from build123d import *

# Parameters (mm, degrees)
SKETCH1_W               = 44.5
SKETCH1_H               = 35
BOSS_EXTRUDE1_DEPTH     = 4
BOSS_EXTRUDE2_DEPTH     = 19.6
SKETCH4_W               = 26
SKETCH4_H               = 31
CUT_EXTRUDE1_DEPTH      = 4
BOSS_EXTRUDE3_DEPTH     = 4
CHAMFER1_SIZE           = 5
CUT_EXTRUDE2_DEPTH      = 62.336856783
CUT_EXTRUDE2_DEPTH_BACK = 62.336856783
SKETCH6_R               = 1.25
SKETCH7_R               = 2.5
SKETCH7_R_2             = 1.25
BOSS_EXTRUDE4_DEPTH     = 4
FILLET1_R               = 0.5
FILLET3_R               = 0.25
CUT_EXTRUDE3_DEPTH      = 60.911685095
CUT_EXTRUDE3_DEPTH_BACK = 60.911685095
SKETCH8_R               = 1.25


with BuildPart() as part:
    # Sketch1 → Boss-Extrude1 (new body)
    with BuildSketch(Plane(origin=(0, 0, 0), x_dir=(1, 0, 0), z_dir=(0, 1, 0))):
        with Locations((22.25, 17.5)):
            Rectangle(SKETCH1_W, SKETCH1_H)
    extrude(amount=BOSS_EXTRUDE1_DEPTH)

    # Sketch3 → Boss-Extrude2 (add)
    with BuildSketch(Plane(origin=(0, 0, 0), x_dir=(1, 0, 0), z_dir=(0, 1, 0))):
        Polygon((9.1, 31), (9.1, 0), (5.1, 0), (5.1, 35), (39.1, 35), (39.1, 0), (35.1, 0), (35.1, 31), align=None)
    extrude(amount=BOSS_EXTRUDE2_DEPTH)

    # Sketch4 → Cut-Extrude1 (cut)
    with BuildSketch(Plane(origin=(0, 4, 0), x_dir=(1, 0, 0), z_dir=(0, 1, 0))):
        with Locations((22.1, 15.5)):
            Rectangle(SKETCH4_W, SKETCH4_H)
    extrude(amount=-CUT_EXTRUDE1_DEPTH, mode=Mode.SUBTRACT)

    # Sketch5 → Boss-Extrude3 (add)
    with BuildSketch(Plane(origin=(0, 19.6, 0), x_dir=(1, 0, 0), z_dir=(0, 1, 0))):
        Polygon((15.85, 0), (5.1, 0), (5.1, 35), (39.1, 35), (39.1, 0), (28.35, 0), (28.35, 7.277215151), (35.065893154, 7.277215151), (35.065893154, 27.5), (9.134106846, 27.5), (9.134106846, 7.277215151), (15.85, 7.277215151), align=None)
    extrude(amount=BOSS_EXTRUDE3_DEPTH)

    # Chamfer1
    chamfer1_edges = [part.edges().sort_by_distance(p)[0] for p in [
        (15.85, 21.6, 0),
        (28.35, 21.6, 0),
    ]]
    chamfer(chamfer1_edges, length=CHAMFER1_SIZE)

    # Sketch6 → Cut-Extrude2 (cut, two sides: drawn at the far end of the back side and taken through both)
    with BuildSketch(Plane(origin=(0, 23.6, 0), x_dir=(1, 0, 0), z_dir=(0, 1, 0)).offset(-CUT_EXTRUDE2_DEPTH_BACK)):
        with Locations(Location((11.85, 4.027215151, 0), (0, 0, 270))):
            Circle(SKETCH6_R)
        with Locations(Location((32.35, 4.027215151, 0), (0, 0, 270))):
            Circle(SKETCH6_R)
        with BuildLine():
            ThreePointArc((11.137729662, 27.5), (11.85, 27.277215151), (12.562270338, 27.5))
            Line((12.562270338, 27.5), (11.137729662, 27.5))
        make_face()
        with BuildLine():
            Line((11.137729662, 27.5), (12.562270338, 27.5))
            ThreePointArc((12.562270338, 27.5), (12.957438017, 27.947490182), (13.1, 28.527215151))
            ThreePointArc((13.1, 28.527215151), (11.270275032, 29.634653168), (11.137729662, 27.5))
        make_face()
        with BuildLine():
            ThreePointArc((33.062270338, 27.5), (33.457438017, 27.947490182), (33.6, 28.527215151))
            ThreePointArc((33.6, 28.527215151), (31.770275032, 29.634653168), (31.637729662, 27.5))
            Line((31.637729662, 27.5), (33.062270338, 27.5))
        make_face()
        with BuildLine():
            Line((33.062270338, 27.5), (31.637729662, 27.5))
            ThreePointArc((31.637729662, 27.5), (32.35, 27.277215151), (33.062270338, 27.5))
        make_face()
    extrude(amount=CUT_EXTRUDE2_DEPTH + CUT_EXTRUDE2_DEPTH_BACK, mode=Mode.SUBTRACT)

    # Sketch7 → Boss-Extrude4 (add)
    # profile 1 of 2: a face of its own
    with BuildSketch(Plane(origin=(0, 23.6, 0), x_dir=(1, 0, 0), z_dir=(0, 1, 0))):
        with Locations((11.85, 28.527215151)):
            Circle(SKETCH7_R)
        with Locations(Location((11.85, 28.527215151, 0), (0, 0, 270))):
            Circle(SKETCH7_R_2, mode=Mode.SUBTRACT)
    # profile 2 of 2: a face of its own
    with BuildSketch(Plane(origin=(0, 23.6, 0), x_dir=(1, 0, 0), z_dir=(0, 1, 0))):
        with Locations((32.35, 28.527215151)):
            Circle(SKETCH7_R)
        with Locations(Location((32.35, 28.527215151, 0), (0, 0, 270))):
            Circle(SKETCH7_R_2, mode=Mode.SUBTRACT)
    extrude(amount=-BOSS_EXTRUDE4_DEPTH)

    # Fillet1
    # the kernel refuses this fillet: 0.5 mm, written as the material it adds along each edge
    with BuildSketch(Plane(origin=(35.065893154, 19.6, -27.5), x_dir=(0, 0, 1), z_dir=(0, 1, 0)), Plane(origin=(9.134106846, 19.6, -27.5), x_dir=(1, 0, 0), z_dir=(0, 1, 0))) as fillet1_piece_1:
        with BuildLine():
            CenterArc((FILLET1_R, -FILLET1_R), FILLET1_R, 90, 90)
            Line((0, -FILLET1_R), (0, 0))
            Line((0, 0), (FILLET1_R, 0))
        make_face()
    extrude(amount=4)
    with BuildSketch(Plane(origin=(34.629216759, 19.6, -27.5), x_dir=(1, 0, 0), z_dir=(0, 1, 0))) as fillet1_piece_2:
        with BuildLine():
            CenterArc((0.30295556, -0.5), FILLET1_R, 90, 59.397982961)
            ThreePointArc((-0.127406493, -0.245464142), (-0.060306377, -0.124495193), (0, 0))
            Line((0, 0), (0.30295556, 0))
        make_face()
    extrude(amount=4)
    with BuildSketch(Plane(origin=(9.570783241, 19.6, -27.5), x_dir=(0.46068413755870835, 0, 0.8875641528372973), z_dir=(0, 1, 0))) as fillet1_piece_3:
        with BuildLine():
            CenterArc((0.304215256, -0.499234564), FILLET1_R, 93.170754575, 59.397982961)
            Line((-0.139566821, -0.268892495), (0, 0))
            ThreePointArc((0, 0), (0.138279662, -0.003827182), (0.276559323, 0))
        make_face()
    extrude(amount=4)

    # Fillet3
    fillet3_edges = [part.edges().sort_by_distance(p)[0] for p in [
        (34.749032737, 21.6, -27.465252505),
        (9.450967263, 21.6, -27.465252505),
    ]]
    fillet(fillet3_edges, radius=FILLET3_R)

    # Sketch8 → Cut-Extrude3 (cut, two sides: drawn at the far end of the back side and taken through both)
    with BuildSketch(Plane(origin=(0, 4, 0), x_dir=(1, 0, 0), z_dir=(0, 1, 0)).offset(-CUT_EXTRUDE3_DEPTH_BACK)):
        with Locations(Location((2.55, 32, 0), (0, 0, 270))):
            Circle(SKETCH8_R)
        with Locations(Location((41.65, 32, 0), (0, 0, 90))):
            Circle(SKETCH8_R)
        with Locations(Location((2.55, 3, 0), (0, 0, 270))):
            Circle(SKETCH8_R)
        with Locations(Location((41.65, 3, 0), (0, 0, 90))):
            Circle(SKETCH8_R)
    extrude(amount=CUT_EXTRUDE3_DEPTH + CUT_EXTRUDE3_DEPTH_BACK, mode=Mode.SUBTRACT)


solid = part.part
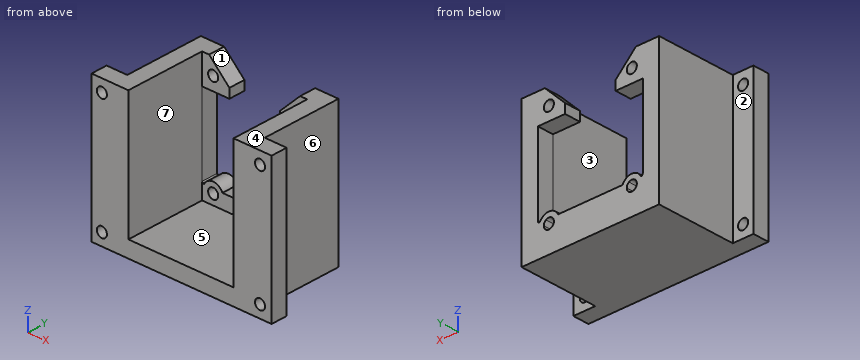
Can you work these out from the model? Positions are in its coordinate system, mm. Face numbers are marked on the shaded views. A direction names the side the tool comes from. Give positions to 0.01 mm unless a question says otherwise; leave off trailing zeros. Loops run counter-clockwise (first coordinate to the right, second up) from the corner with the lowest first, then second, coordinate; pieces in that order, holes last. Notation, with made-up numbers: (-19, 19.25) - (26, 19.25) arc R24 ccw to (26, 54.25) - close; hole circle Ø4 at (7, 32). An arc over 180 degrees is marked (long way). Return JSON: item names as keys, results as strings.
1. For the marked faces 1, 2 and 3, which set-ups out of +Z, -Z, +X, -X, +Y, -Y let a thin tool reach every point of the face, with its end or its side?
Output values:
{"face 1": "+Z, +Y, -Y", "face 2": "+Z, -Z, -X, +Y", "face 3": "+Z, -Y"}
2. I want a section at D-D on x = 11.85. Please give me the cut outline in (y, z).
Output values:
{"outline": "(0, -35) - (23.6, -35) - (23.6, -29.78) - (19.6, -29.78) - (19.6, -31) - (0, -31) - close; (19.6, -27.28) - (23.6, -27.28) - (23.6, -26.03) - (19.6, -26.03) - close; (19.6, -7.28) - (23.6, -7.28) - (23.6, -5.28) - (19.6, -5.28) - close; (19.6, -2.78) - (23.6, -2.78) - (23.6, -1) - (19.6, -1) - close"}
3. I'm going to push flat-ended pins straight in: pin 1 Ø4 at (y, z) = (18, -18) entering from +X; pin 2 Ø3 at (x, z) = (41.65, -32) entering from -Y; pin 3 Ø3 at (x, z) = (2.55, -3) entering from +Y; pin 4 Ø2 at (y, z) = (21, -18) entering from -X. Where does each tip first touch, or does it pass through?
Output values:
{"pin 1": "stops at x = 39.1", "pin 2": "stops at y = 0", "pin 3": "stops at y = 4", "pin 4": "stops at x = 5.1"}
4. If I drill on line 1 (X direction, y = 3.15, z = -3); line 2 (X direction, y = 2.7, z = -32); line 3 (X direction, y = 15.25, z = -11), over which ranges is the centre line in solid material (lowest first)?
Output values:
{"line 1": "x = 0 to 1.3, 3.8 to 9.1, 35.1 to 40.4, 42.9 to 44.5", "line 2": "x = 0 to 1.3, 3.8 to 40.4, 42.9 to 44.5", "line 3": "x = 5.1 to 9.1, 35.1 to 39.1"}
5. We'd pull the mould along X, two halves only. Please class the marked faces 4, 5, 6 and 7: +X half, -X half, draft (parallel to the pull), parting line (faces both ways), or undercut.
Output values:
{"face 4": "draft", "face 5": "undercut", "face 6": "+X half", "face 7": "undercut"}
6. I want a section at B-B on x = 2.55. Please give me the cut outline in (y, z), and give its area (3 significant figures).
Output values:
{"outline": "(0, -35) - (4, -35) - (4, -33.25) - (0, -33.25) - close; (0, -30.75) - (4, -30.75) - (4, -4.25) - (0, -4.25) - close; (0, -1.75) - (4, -1.75) - (4, 0) - (0, 0) - close", "area": "120 mm²"}
7. I want a section at A-A on z = -32. Please give me the cut outline in (x, y).
Output values:
{"outline": "(0, 0) - (1.3, 0) - (1.3, 4) - (0, 4) - close; (3.8, 0) - (40.4, 0) - (40.4, 4) - (39.1, 4) - (39.1, 23.6) - (5.1, 23.6) - (5.1, 4) - (3.8, 4) - close; (42.9, 0) - (44.5, 0) - (44.5, 4) - (42.9, 4) - close"}
